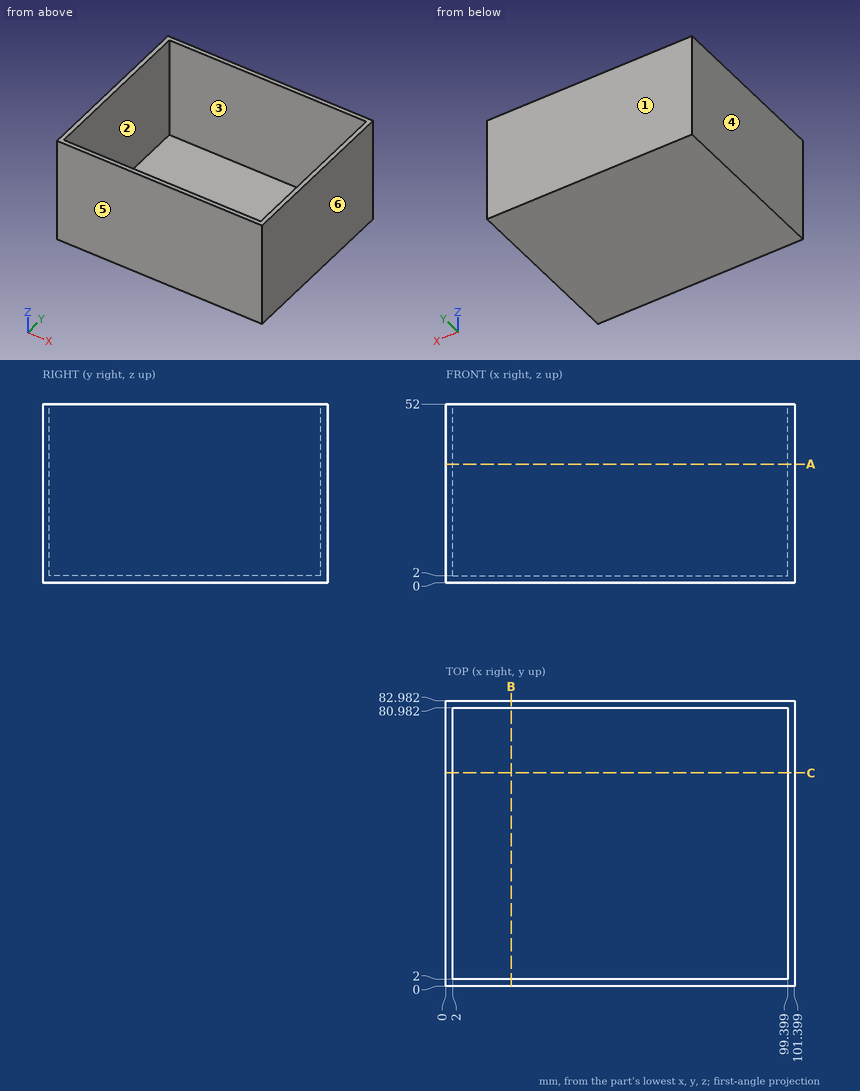
Check sheet for the drawn part. Datum: minimum x, y, z corner. Units: mm. A direction names the side the tool comes from. Round coordinates to 2 decimals unless told otherwise and drop trailing zeros. Order: outer loops, then holes, each group sorted by start corner. A loop starts at its lowest first (then second) coordinate and runs counter-clockwise, first axis right, second up.
1. Section check B-B on x = 19. Record the cut outline in (y, z), then the cut area to 3 significant figures.
Final values:
outline: (0, 0) - (82.98, 0) - (82.98, 52) - (80.98, 52) - (80.98, 2) - (2, 2) - (2, 52) - (0, 52) - close
area: 366 mm2
2. Thickness scan on L1, parallel to X at y = 60, z = 32; L2, parallel to Y at x = 67.5, z = 6; L3, parallel to Z at x = 31.5, y = 59. Record the ranges inside material, lowest first.
Final values:
L1: x = 0 to 2, 99.4 to 101.4
L2: y = 0 to 2, 80.98 to 82.98
L3: z = 0 to 2
3. Go/stop test with a flat-tipped pin: P1, Ø8, axis at x = 37.5, y = 61.5, coming from the +Z side. Record where the tip stops, or that it passes through.
Final values:
P1: stops at z = 2
4. Section check C-C on y = 62. Record the cut outline in (x, z), then the cut area to 3 significant figures.
Final values:
outline: (0, 0) - (101.4, 0) - (101.4, 52) - (99.4, 52) - (99.4, 2) - (2, 2) - (2, 52) - (0, 52) - close
area: 403 mm2
5. Section check A-A on z = 34.5. Record the cut outline in (x, y).
Final values:
outline: (0, 0) - (101.4, 0) - (101.4, 82.98) - (0, 82.98) - close; hole (2, 2) - (99.4, 2) - (99.4, 80.98) - (2, 80.98) - close
6. Access from +Z, -Z, +X, -X, +Y, -Y to the whole of each face (thin tool, end or side, straight path). Record for the marked faces 1 and 2.
Final values:
face 1: +Z, -Z, +X, -X, +Y
face 2: +Z
7. Release check for a two-part mould opening along X. For the marked faces 3, 4, 5 and 6 record: +X half, -X half, draft (parallel to the pull), parting line (faces both ways), or undercut.
Final values:
face 3: undercut
face 4: -X half
face 5: draft
face 6: +X half
